Verification items for the finished model (mm, model axes). Face numbers are marked on the shaded views. A direction names the side the tool comes from. Give positions to 0.01 mm unless a question says otherwise; leave off trailing zeros. Write each loop counter-clockwise with the first axis right and the second up, starting at its lowest first coordinate (ties: lowest second). Pieces come first, ordered by that corner, then holes. Notation, with made-up numbers: M 88.25,26 L 103.25,26 A35 ccw 103.25,65 Z; hole C 41,64 d7. An arc over 180 degrees is marked long. Answer as a JSON object with one key per item and string values.
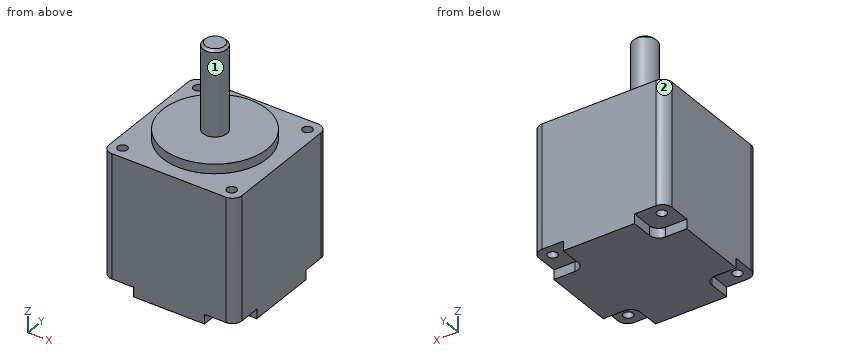
Autodesk Inventor part; units mm, degrees
ref_plane "YZ Plane" through (0, 0, 0) normal (1, 0, 0) x (0, 1, 0)
ref_plane "XZ Plane" through (0, 0, 0) normal (0, 1, 0) x (-1, 0, 0)
ref_plane "XY Plane" through (0, 0, 0) normal (0, 0, 1) x (1, 0, 0)
sketch "Sketch6" plane through (0, 0, 0) normal (0, 0, 1) x (1, 0, 0)
  line L0 (20.7414, 11.7807) -> (48.7414, 11.7807)
  line L1 (48.7414, 11.7807) -> (48.7414, -16.2193)
  line L2 (48.7414, -16.2193) -> (20.7414, -16.2193)
  line L3 (20.7414, -16.2193) -> (20.7414, 11.7807)
  point P0 (0, 0)
  dimension "d10" = 28
extrude "Extrusion6" add sketch "Sketch6" against normal blind 28
sketch "Sketch7" plane through (0, 0, 0) normal (0, 0, 1) x (1, 0, 0)
  line L0 (48.7414, 11.7807) -> (20.7414, 11.7807)
  line L1 (20.7414, 11.7807) -> (20.7414, -16.2193)
  line L2 (48.7414, -16.2193) -> (48.7414, 11.7807)
  line L3 (20.7414, -16.2193) -> (48.7414, -16.2193)
  point P0 (0, 0)
  point P1 (23.2414, 9.2807)
  point P2 (46.2414, 9.2807)
  point P3 (46.2414, -13.7193)
  point P4 (23.2414, -13.7193)
  point P5 (46.7414, 11.7807)
  point P6 (22.7414, 11.7807)
  point P7 (20.7414, 9.7807)
  point P8 (20.7414, -14.2193)
  point P9 (48.7414, -14.2193)
  point P10 (48.7414, 9.7807)
  point P11 (22.7414, -16.2193)
  point P12 (46.7414, -16.2193)
  dimension "d14" = 2.5
  dimension "d15" = 2.5
  dimension "d16" = 2.5
  dimension "d17" = 2.5
hole "Hole1" at (23.2414, 9.2807, 0) at (46.2414, 9.2807, 0) at (46.2414, -13.7193, 0) at (23.2414, -13.7193, 0) direction (0, 0, -1) diameter 2.013 depth 4.5
sketch "Sketch8" plane through (0, 0, 0) normal (0, 0, 1) x (1, 0, 0)
  circle A0 centre (34.7414, -2.2193) radius 11
  line L0 (48.7414, -16.2193) -> (48.7414, 11.7807)
  line L1 (48.7414, 11.7807) -> (20.7414, 11.7807)
  point P0 (0, 0)
  point P1 (48.7414, -2.2193)
  point P2 (48.7414, -14.2193)
  point P3 (48.7414, 9.7807)
  point P4 (34.7414, 11.7807)
  point P5 (46.7414, 11.7807)
  point P6 (22.7414, 11.7807)
  dimension "d25" = 22
extrude "Extrusion7" add sketch "Sketch8" along normal blind 2
sketch "Sketch9" plane through (34.7414, -2.2193, 2) normal (0, 0, 1) x (1, 0, 0)
  circle A0 centre (0, 0) radius 2.5
  circle A1 centre (0, 0) radius 11
  point P0 (-34.7414, 2.2193)
  dimension "d28" = 5
extrude "Extrusion8" add sketch "Sketch9" along normal blind 18 contours A0
chamfer "Chamfer1" distance 0.5 angle 45 1 edges at (32.2414, -2.2193, 20)
sketch "Sketch10" plane through (0, 0, -28) normal (0, 0, -1) x (-1, 0, 0)
  line L0 (-20.7414, 11.7807) -> (-27.2414, 11.7807)
  line L1 (-27.2414, 11.7807) -> (-27.2414, 5.2807)
  line L2 (-27.2414, 5.2807) -> (-20.7414, 5.2807)
  line L3 (-20.7414, 5.2807) -> (-20.7414, 11.7807)
  line L4 (-20.7414, -16.2193) -> (-27.2414, -16.2193)
  line L5 (-27.2414, -16.2193) -> (-27.2414, -9.7193)
  line L6 (-27.2414, -9.7193) -> (-20.7414, -9.7193)
  line L7 (-20.7414, -9.7193) -> (-20.7414, -16.2193)
  line L8 (-48.7414, -16.2193) -> (-42.2414, -16.2193)
  line L9 (-42.2414, -16.2193) -> (-42.2414, -9.7193)
  line L10 (-42.2414, -9.7193) -> (-48.7414, -9.7193)
  line L11 (-48.7414, -9.7193) -> (-48.7414, -16.2193)
  line L12 (-42.2414, 11.7807) -> (-48.7414, 11.7807)
  line L13 (-48.7414, 11.7807) -> (-48.7414, 5.2807)
  line L14 (-48.7414, 5.2807) -> (-42.2414, 5.2807)
  line L15 (-42.2414, 5.2807) -> (-42.2414, 11.7807)
  line L16 (-20.7414, -16.2193) -> (-20.7414, 11.7807)
  line L17 (-20.7414, 11.7807) -> (-48.7414, 11.7807)
  line L18 (-48.7414, -16.2193) -> (-20.7414, -16.2193)
  line L19 (-48.7414, 11.7807) -> (-48.7414, -16.2193)
  point P0 (0, 0)
  point P1 (-20.7414, -14.2193)
  point P2 (-20.7414, 9.7807)
  point P3 (-22.7414, 11.7807)
  point P4 (-46.7414, 11.7807)
  point P5 (-46.7414, -16.2193)
  point P6 (-22.7414, -16.2193)
  point P7 (-48.7414, 9.7807)
  point P8 (-48.7414, -14.2193)
  dimension "d34" = 6.5
extrude "Extrusion9" cut sketch "Sketch10" against normal blind 2 contours L3 L2 L1 L0 | L15 L14 L13 L12 | L7 L4 L5 L6 | L10 L9 L8 L11
sketch "Sketch11" plane through (0, 0, -26) normal (0, 0, -1) x (-1, 0, 0)
  circle A0 centre (-23.2414, -13.7193) radius 1.0065
  circle A1 centre (-23.2414, 9.2807) radius 1.0065
  circle A2 centre (-46.2414, -13.7193) radius 1.0065
  circle A3 centre (-46.2414, 9.2807) radius 1.0065
  point P0 (0, 0)
extrude "Extrusion10" cut sketch "Sketch11" against normal blind 4.5
fillet "Fillet2" radius 2 8 edges at (20.7414, 11.7807, -13) (48.7414, 11.7807, -13) (20.7414, -16.2193, -13) (48.7414, -16.2193, -13) (27.2414, -9.7193, -27) (27.2414, 5.2807, -27) (42.2414, 5.2807, -27) (42.2414, -9.7193, -27)
equation "\"d11\" = MotorHeightBase"
equation "\"MotorHeightBase\" = 28"
properties part number "NEMA 11"
1) Section check B-B on x = 25.75. Record the boundary of the cut face in (y, z).
Completed:
{"outline": "M -16.22,-26 L -9.79,-26 L -9.79,-28 L 5.35,-28 L 5.35,-26 L 11.78,-26 L 11.78,0 L 4.12,0 L 4.12,2 L -8.56,2 L -8.56,0 L -16.22,0 Z"}
2) Thickness scan on L1, parallel to Z at x = 32.75, y = 1; L2, parallel to Z at x = 22.5, y = 2.5; L3, parallel to Y at x = 23, z = -1. Record the ranges inside material, lowest first.
Completed:
{"L1": "z = -28 to 2", "L2": "z = -28 to 0", "L3": "y = -16.22 to -14.7, -12.74 to 8.3, 10.26 to 11.78"}
3) Section check C-C on z = -24. Record the boundary of the cut face in (x, y).
Completed:
{"outline": "M 20.74,-14.22 A2 ccw 22.74,-16.22 L 46.74,-16.22 A2 ccw 48.74,-14.22 L 48.74,9.78 A2 ccw 46.74,11.78 L 22.74,11.78 A2 ccw 20.74,9.78 Z; hole C 23.24,-13.72 d2.01; hole C 23.24,9.28 d2.01; hole C 46.24,-13.72 d2.01; hole C 46.24,9.28 d2.01"}
4) Section check D-D on z = 0.5. Record the boundary of the cut face in (x, y), and give its area (3 significant figures).
Completed:
{"outline": "C 34.74,-2.22 d22", "area": "380 mm2"}
5) Go/stop test with flat-tipped pins: pin 1 (0.6 mm diameter, centred on y = -13.5, z = -27.5, fed in from -X); pin 2 (1.2 mm diameter, centred on x = 23.24, y = -13.72, fed in from -Z); pin 3 (2 mm diameter, centred on x = 46, y = 9.5, fed in from -Z). Record where each tip stops, or that it passes through.
Completed:
{"pin 1": "stops at x = 27.24", "pin 2": "stops at z = -21.5", "pin 3": "stops at z = -26"}
6) Access from +Z, -Z, +X, -X, +Y, -Y to the whole of each face (thin tool, end or side, straight path). Record for the marked faces 1 and 2.
Completed:
{"face 1": "+Z", "face 2": "+Z, -Z, -X, +Y"}
7) Section check A-A on y = -9. Record the boundary of the cut face in (x, z).
Completed:
{"outline": "M 20.74,-28 L 48.74,-28 L 48.74,0 L 43.4,0 L 43.4,2 L 26.08,2 L 26.08,0 L 20.74,0 Z"}
